Input: part model. Units: mm. Frame: model coordinates. Round coordinates to 2 decimals unless told otherwise and drop trailing zeros. Loops run counter-clockwise (first coordinate to the right, second up) from the corner with the lowest first, then second, coordinate; pieces in that order, holes last. Notation, with made-up numbers: M 1,19.25 L 48,19.25 A33 ccw 48,54.25 Z; hole C 36.5,70.25 d2. An arc over 180 degrees is marked long. Use one line per item in the form item = value. Start each with the question number.
Q1. Ray query, line 1 along X through (y, z) = (-2.5, 6); line 2 along Y through (x, z) = (208, 5) (3 decimals); line 3 along X through (y, z) = (-7.5, 9.75). Return the intervals inside material, ascending.
Q2. Section query B-B, the plane x = 220.5. Output: boundary loops of the cut face in (y, z) (3 decimals), and give its area (3 significant figures).
Q3. Section query C-C, the plane y = -41.5. Output: boundary loops of the cut face in (x, z).
Q4. Section query D-D, the plane y = 41. Output: boundary loops of the cut face in (x, z).
Q5. First-contact query: P1, Ø8, axis at y = -16, z = 7, coming from the +X side; P2, Ø4, axis at y = 8, z = 15.5, coming from the +X side. Flat tips, straight axial feed; report the tip coordinate or a pass-through.
Q6. Section query A-A, the plane y = 0. Output: boundary loops of the cut face in (x, z) (3 decimals).
```python
from build123d import *

# Parameters (mm, degrees)
F2_DEPTH = 19.05


# Not quite as in the source:
# - a variable given as a bare number and used for a length is read in inches; the dataset says mm whatever the document's units were


with BuildPart() as f2:
    # F1 (on Top) → F2 (new body)
    with BuildSketch(Plane.XY):
        with BuildLine():
            Line((234.95, 47.625), (-234.95, 47.625))
            Line((-234.95, 47.625), (-234.95, 18.5052561211))
            ThreePointArc((-234.95, 18.5052561211), (-230.3478700667, 15.024261314), (-228.6, 9.525))
            Line((-228.6, 9.525), (-177.8, 9.525))
            ThreePointArc((-177.8, 9.525), (-168.275, 19.05), (-158.75, 9.525))
            Line((-158.75, 9.525), (-158.75, -9.525))
            ThreePointArc((-158.75, -9.525), (-168.275, -19.05), (-177.8, -9.525))
            Line((-177.8, -9.525), (-228.6, -9.525))
            ThreePointArc((-228.6, -9.525), (-230.3478700667, -15.024261314), (-234.95, -18.5052561211))
            Line((-234.95, -18.5052561211), (-234.95, -47.625))
            Line((-234.95, -47.625), (234.95, -47.625))
            Line((234.95, -47.625), (234.95, -18.5052561211))
            ThreePointArc((234.95, -18.5052561211), (230.3478700667, -15.024261314), (228.6, -9.525))
            Line((228.6, -9.525), (177.8, -9.525))
            ThreePointArc((177.8, -9.525), (168.275, -19.05), (158.75, -9.525))
            Line((158.75, -9.525), (158.75, 9.525))
            ThreePointArc((158.75, 9.525), (168.275, 19.05), (177.8, 9.525))
            Line((177.8, 9.525), (228.6, 9.525))
            ThreePointArc((228.6, 9.525), (230.3478700667, 15.024261314), (234.95, 18.5052561211))
            Line((234.95, 18.5052561211), (234.95, 47.625))
        make_face()
        with BuildLine():
            Line((-234.95, 18.5052561211), (-234.95, 47.625))
            ThreePointArc((-234.95, 47.625), (-282.575, 0), (-234.95, -47.625))
            Line((-234.95, -47.625), (-234.95, -18.5052561211))
            ThreePointArc((-234.95, -18.5052561211), (-243.624261314, -17.3021299333), (-247.65, -9.525))
            Line((-247.65, -9.525), (-247.65, 9.525))
            ThreePointArc((-247.65, 9.525), (-243.624261314, 17.3021299333), (-234.95, 18.5052561211))
        make_face()
        with BuildLine():
            ThreePointArc((234.95, -47.625), (282.575, 0), (234.95, 47.625))
            Line((234.95, 47.625), (234.95, 18.5052561211))
            ThreePointArc((234.95, 18.5052561211), (243.624261314, 17.3021299333), (247.65, 9.525))
            Line((247.65, 9.525), (247.65, -9.525))
            ThreePointArc((247.65, -9.525), (243.624261314, -17.3021299333), (234.95, -18.5052561211))
            Line((234.95, -18.5052561211), (234.95, -47.625))
        make_face()
    extrude(amount=F2_DEPTH)


solid = f2.part
```
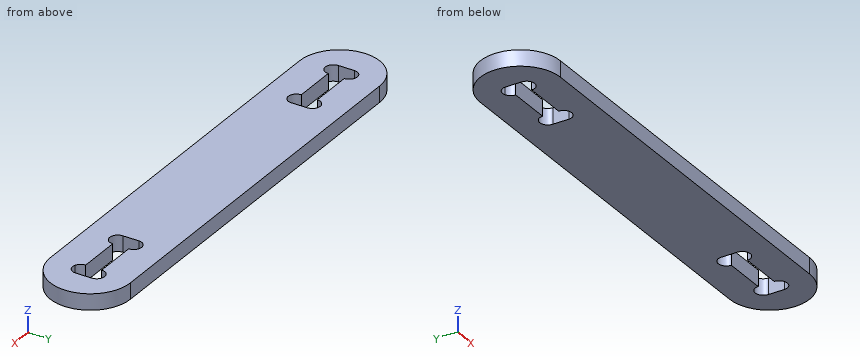
Results found:
q1.line_1 = -282.51 to -247.65, -158.75 to 158.75, 247.65 to 282.51
q1.line_2 = -47.625 to -9.525, 9.525 to 47.625
q1.line_3 = -281.98 to -247.65, -158.75 to 158.75, 247.65 to 281.98
q2.outline = M -47.625,0 L -9.525,0 L -9.525,19.05 L -47.625,19.05 Z; M 9.525,0 L 47.625,0 L 47.625,19.05 L 9.525,19.05 Z
q2.area = 1,450 mm²
q3.outline = M -258.31,0 L 258.31,0 L 258.31,19.05 L -258.31,19.05 Z
q4.outline = M -259.18,0 L 259.18,0 L 259.18,19.05 L -259.18,19.05 Z
q5.P1 = 281.04
q5.P2 = 282.2
q6.outline = M -282.575,0 L -247.65,0 L -247.65,19.05 L -282.575,19.05 Z; M -158.75,0 L 158.75,0 L 158.75,19.05 L -158.75,19.05 Z; M 247.65,0 L 282.575,0 L 282.575,19.05 L 247.65,19.05 Z
